from build123d import *

# Parameters (mm, degrees)
SKETCH_2_W          = 19
SKETCH_2_H          = 31.7
EXTRUDE_1_DEPTH     = 6.6
SKETCH_3_W          = 19
SKETCH_3_H          = 38
EXTRUDE_2_DEPTH     = 6.6
SKETCH_4_W          = 8.1
SKETCH_4_H          = 25.10428036
EXTRUDE_3_DEPTH     = 2
SKETCH_5_W          = 8.1
SKETCH_5_H          = 24
EXTRUDE_4_DEPTH     = 2
SKETCH_6_W          = 5.45
SKETCH_6_H          = 7.386023797
SKETCH_6_H_2        = 7.397863342
CUT_EXTRUDE_1_DEPTH = 42.306415967
CHAMFER_1_SIZE      = 5
SKETCH_7_R          = 3
CUT_EXTRUDE_2_DEPTH = 35.725098992
SKETCH_8_R          = 3
CUT_EXTRUDE_3_DEPTH = 41.122562231
SKETCH_9_W          = 5.45
SKETCH_9_H          = 2
CUT_EXTRUDE_4_DEPTH = 25
CUT_EXTRUDE_5_DEPTH = 35.725098992


with BuildPart() as part:
    # 草图2 → 凸台-拉伸1 (new body)
    with BuildSketch(Plane.XY):
        Rectangle(SKETCH_2_W, SKETCH_2_H)
    extrude(amount=EXTRUDE_1_DEPTH)

    # 草图3 → 凸台-拉伸2 (add)
    with BuildSketch(Plane(origin=(0, 15.85, 0), x_dir=(1, 0, 0), z_dir=(0, 1, 0))):
        with Locations((0, 12.4)):
            Rectangle(SKETCH_3_W, SKETCH_3_H)
    extrude(amount=-EXTRUDE_2_DEPTH)

    # 草图4 → 凸台-拉伸3 (add)
    with BuildSketch(Plane(origin=(0, 0, 0), x_dir=(-1, 0, 0), z_dir=(0, 0, -1))):
        with Locations((0, -3.29785982)):
            Rectangle(SKETCH_4_W, SKETCH_4_H)
    extrude(amount=EXTRUDE_3_DEPTH)

    # 草图5 → 凸台-拉伸4 (add)
    with BuildSketch(Plane.XZ.offset(-9.25)):
        with Locations((0, -19.4)):
            Rectangle(SKETCH_5_W, SKETCH_5_H)
    extrude(amount=EXTRUDE_4_DEPTH)

    # 草图6 → 切除-拉伸1 (cut, through all)
    with BuildSketch(Plane.XZ.offset(-9.25)):
        with Locations((-6.775, -3.706988102)):
            Rectangle(SKETCH_6_W, SKETCH_6_H)
        with Locations((6.775, -3.701068329)):
            Rectangle(SKETCH_6_W, SKETCH_6_H_2)
    extrude(amount=-CUT_EXTRUDE_1_DEPTH, mode=Mode.SUBTRACT)

    # 倒角1
    chamfer_1_edges = [part.edges().sort_by_distance(p)[0] for p in [
        (-9.5, 0, 6.6),
        (9.5, 0, 6.6),
    ]]
    chamfer(chamfer_1_edges, length=CHAMFER_1_SIZE)

    # 草图7 → 切除-拉伸2 (cut, through all)
    with BuildSketch(Plane(origin=(0, 0, -2), x_dir=(-1, 0, 0), z_dir=(0, 0, -1))):
        with Locations((0, -4.859710354)):
            Circle(SKETCH_7_R)
    extrude(amount=-CUT_EXTRUDE_2_DEPTH, mode=Mode.SUBTRACT)

    # 草图8 → 切除-拉伸3 (cut, through all)
    with BuildSketch(Plane.XZ.offset(-7.25)):
        with Locations(Location((0, -19.674028048, 0), (0, 0, 270))):
            Circle(SKETCH_8_R)
    extrude(amount=-CUT_EXTRUDE_3_DEPTH, mode=Mode.SUBTRACT)

    # 草图9 → 切除-拉伸4 (cut)
    with BuildSketch(Plane(origin=(0, 0, -31.4), x_dir=(-1, 0, 0), z_dir=(0, 0, -1))):
        with Locations((-6.775, 14.85)):
            Rectangle(SKETCH_9_W, SKETCH_9_H)
        with Locations((6.775, 14.85)):
            Rectangle(SKETCH_9_W, SKETCH_9_H)
    extrude(amount=-CUT_EXTRUDE_4_DEPTH, mode=Mode.SUBTRACT)

    # 草图10 → 切除-拉伸5 (cut, through all)
    with BuildSketch(Plane(origin=(0, 0, -2), x_dir=(-1, 0, 0), z_dir=(0, 0, -1))):
        Polygon((-4.05, -15.85), (-9.5, -10.999261641), (-9.5, -15.85), align=None)
    cut_extrude_5 = extrude(amount=-CUT_EXTRUDE_5_DEPTH, mode=Mode.SUBTRACT)

    # 镜向1: 切除-拉伸5 across plane
    add(cut_extrude_5.mirror(Plane(origin=(0, 0, 0), x_dir=(0, 0, 1), z_dir=(1, 0, 0))), mode=Mode.SUBTRACT)


solid = part.part
Geometry check sheet. Reference: the model listing, model coordinates, mm. A direction names the side the tool comes from. Coordinates: 2 decimals unless noted, no trailing zeros. Write each loop counter-clockwise with the first axis right and the second up, starting at its lowest first coordinate (ties: lowest second). Pieces come first, ordered by that corner, then holes. Notation, with made-up numbers: (79, 62.25) -> (105, 62.25) arc R5 cw to (105, 67.25) -> close; hole circle Ø9 at (-8.75, -26). An arc over 180 degrees is marked (long way). One line per question, with ' | ' between items.
1. Cross-section at B-B on y = -7. Record the cut outline in (x, z), and give its area (3 significant figures).
Answers:
outline: (-9.5, 0) -> (-4.05, 0) -> (-4.05, -2) -> (-2.1, -2) -> (-2.1, 6.6) -> (-4.5, 6.6) -> (-9.5, 1.6) -> close; (2.1, -2) -> (4.05, -2) -> (4.05, 0) -> (9.5, 0) -> (9.5, 1.6) -> (4.5, 6.6) -> (2.1, 6.6) -> close | area: 80.4 mm²
2. Cross-section at D-D on z = -19. Record the cut outline in (x, y).
Answers:
outline: (-9.5, 9.25) -> (-4.05, 9.25) -> (-4.05, 7.25) -> (-2.92, 7.25) -> (-2.92, 15.85) -> (-4.05, 15.85) -> (-4.05, 13.85) -> (-9.5, 13.85) -> close; (2.92, 7.25) -> (4.05, 7.25) -> (4.05, 9.25) -> (9.5, 9.25) -> (9.5, 13.85) -> (4.05, 13.85) -> (4.05, 15.85) -> (2.92, 15.85) -> close
3. Set-up check for faces 5 (the flat face through (7, 9.25, -20)), 6 (the flat face through (0, 8, -7.4)), 7 (the flat face through (-4.05, 8, -20)), 8 (the flat face through (-7, 13.85, -20)), 9 (the flat face through (-7, 12, -7.4)): record each of +Z, -Z, +X, -X, +Y, -Y from which the full face is reachable in a straight line by a thin tool's end or side.
Answers:
face 5: -Z, +X, -Y | face 6: +X, -X, -Y | face 7: -Z, -X, -Y | face 8: -Z, -X, +Y | face 9: -X, +Y, -Y
4. Cross-section at A-A on x = 0. Record the cut outline in (y, z).
Answers:
outline: (-15.85, -2) -> (-7.86, -2) -> (-7.86, 6.6) -> (-15.85, 6.6) -> close; (-1.86, -2) -> (9.25, -2) -> (9.25, -7.4) -> (7.25, -7.4) -> (7.25, -16.67) -> (15.85, -16.67) -> (15.85, 6.6) -> (-1.86, 6.6) -> close; (7.25, -31.4) -> (15.85, -31.4) -> (15.85, -22.67) -> (7.25, -22.67) -> close
5. Thickness scan on probe 1 along Y at (x, z) = (0, 4); probe 2 along Y at (x, z) = (-1, -4); probe 3 along Z at (x, y) = (-1.5, 11). Record the ranges inside material, lowest first. Write a range as from..to.
Answers:
probe 1: y = -15.85..-7.86, -1.86..15.85 | probe 2: y = 9.25..15.85 | probe 3: z = -31.4..-22.27, -17.08..6.6
6. Depth check by flat-ended pin: pin 1 Ø2.5 at (x, z) = (5.5, -24.5) entering from +Y; pin 2 Ø3.5 at (x, y) = (0, -4.86) entering from +Z; pin 3 Ø2.5 at (x, y) = (7, 14) entering from -Z; pin 4 Ø2.5 at (x, z) = (1.5, -6) entering from -Y. Enter the tip coordinate at first touch or a pass-through.
Answers:
pin 1: stops at y = 13.85 | pin 2: passes through | pin 3: stops at z = -31.4 | pin 4: stops at y = 9.25
7. Draft check along Z on faces 1 (the flat face through (-7, -3, 0)), 2 (the flat face through (-7, 0, 4.1)), 3 (the flat face through (4.05, 10, -6)), 4 (the flat face through (6.13, -14, 2.52)). Enter one of: +Z half, -Z half, draft (parallel to the pull), parting line (faces both ways), or undercut.
Answers:
face 1: -Z half | face 2: +Z half | face 3: undercut | face 4: draft
8. Cross-section at C-C on y = 11.5. Record the cut outline in (x, z).
Answers:
outline: (-9.5, -31.4) -> (9.5, -31.4) -> (9.5, -7.4) -> (4.05, -7.4) -> (4.05, 0) -> (9.5, 0) -> (9.5, 1.6) -> (4.5, 6.6) -> (-4.5, 6.6) -> (-9.5, 1.6) -> (-9.5, -0.01) -> (-4.05, -0.01) -> (-4.05, -7.4) -> (-9.5, -7.4) -> close; hole circle Ø6 at (0, -19.67)
